For this review, use the dimensioned drawing (mm, ordinates from the lowest corner) and the shaded views. Coordinates: 2 decimals unless noted, no trailing zeros. Order: outer loops, then holes, each group sorted by start corner. A loop starts at its lowest first (then second) coordinate and runs counter-clockwise, first axis right, second up. Notation, with made-up numbers: M 63.5,53.25 L 95.5,53.25 A19 ccw 95.5,58.25 Z; hole C 39.25,24 d3. An arc over 180 degrees is marked long. One line per item, written item: value.
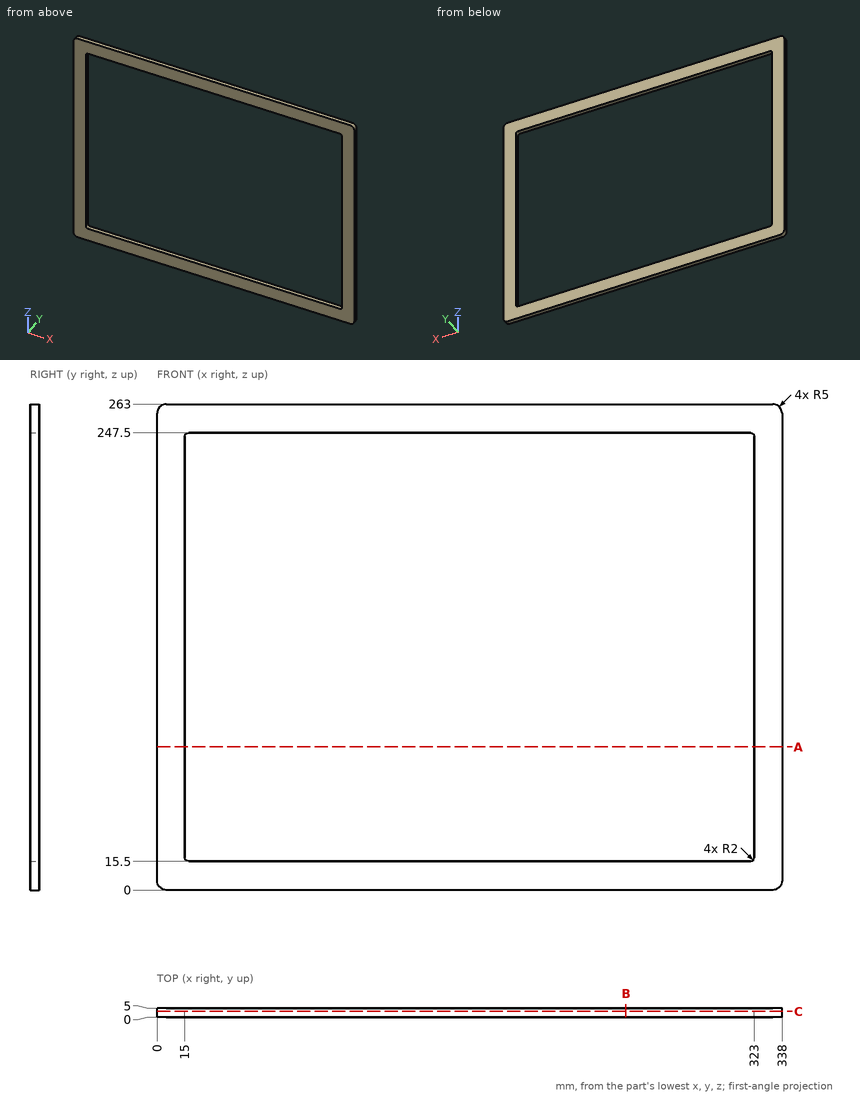
(1) For L1, parallel to X at y = 2.2, z = 133; L2, parallel to Z at x = 196.5, y = 3.45, list the stretches that pass through material, from the lowest coordinate up.
Geometry results:
L1: x = 0 to 15, 323 to 338
L2: z = 0 to 15.5, 247.5 to 263
(2) Insertion check: pin 1 Ø2 at (y, z) = (3, 37) entering from -X. The pin has a flat end and moves straight along its axis. Give the tip position at first contact, or say it passes through.
Geometry results:
pin 1: stops at x = 0
(3) We need section B-B, the plane x = 253.5. State the section outline as (y, z) points.
Geometry results:
outline: M 0,0 L 5,0 L 5,15.5 L 0,15.5 Z; M 0,247.5 L 5,247.5 L 5,263 L 0,263 Z
(4) We need section C-C, the plane y = 3.2. State the section outline as (x, z) points.
Geometry results:
outline: M 0,5 A5 ccw 5,0 L 333,0 A5 ccw 338,5 L 338,258 A5 ccw 333,263 L 5,263 A5 ccw 0,258 Z; hole M 15,17.5 A2 ccw 17,15.5 L 321,15.5 A2 ccw 323,17.5 L 323,245.5 A2 ccw 321,247.5 L 17,247.5 A2 ccw 15,245.5 Z
(5) We need section A-A, the plane z = 77.5. State the section outline as (x, y) points, plus the area to 3 significant figures.
Geometry results:
outline: M 0,0 L 15,0 L 15,5 L 0,5 Z; M 323,0 L 338,0 L 338,5 L 323,5 Z
area: 150 mm2
